from build123d import *

# Parameters (mm, degrees)
CROQUIS1_W              = 8.2
CROQUIS1_H              = 3
CROQUIS1_W_2            = 3
CROQUIS1_H_2            = 7.7
CROQUIS1_W_3            = 40
CROQUIS1_H_3            = 40
SALIENTE_EXTRUIR1_DEPTH = 3


with BuildPart() as part:
    # Croquis1 → Saliente-Extruir1 (new body)
    with BuildSketch(Plane.XY):
        Polygon((-20, 20), (-11.8, 20), (-11.8, 23), (-23, 23), (-23, 20), align=None)
        with Locations((0, 21.5)):
            Rectangle(CROQUIS1_W, CROQUIS1_H)
        Polygon((11.8, 20), (20, 20), (23, 20), (23, 23), (11.8, 23), align=None)
        with Locations((21.5, 7.95)):
            Rectangle(CROQUIS1_W_2, CROQUIS1_H_2)
        with Locations((21.5, -7.95)):
            Rectangle(CROQUIS1_W_2, CROQUIS1_H_2)
        Polygon((23, -20), (20, -20), (11.8, -20), (11.8, -23), (23, -23), align=None)
        with Locations((0, -21.5)):
            Rectangle(CROQUIS1_W, CROQUIS1_H)
        Polygon((-11.8, -23), (-11.8, -20), (-20, -20), (-23, -20), (-23, -23), align=None)
        with Locations((-21.5, 7.95)):
            Rectangle(CROQUIS1_W_2, CROQUIS1_H_2)
        Rectangle(CROQUIS1_W_3, CROQUIS1_H_3)
        with Locations((-21.5, -7.95)):
            Rectangle(CROQUIS1_W_2, CROQUIS1_H_2)
    extrude(amount=SALIENTE_EXTRUIR1_DEPTH)


solid = part.part
Can you work these out from the model? Positions are in its coordinate system, mm. A direction names the side the tool comes from. Coordinates: 2 decimals unless noted, no trailing zeros. Loops run counter-clockwise (first coordinate to the right, second up) from the corner with the lowest first, then second, coordinate; pieces in that order, holes last. Notation, with made-up numbers: (18.25, -9) - (24.25, -9) arc R13 ccw to (24.25, 12) - close; hole circle Ø6 at (44, -5). An arc over 180 degrees is marked (long way). Put each result on its own line as item: value. Start each with the question number.
Item 1: If we mould it in two halves opening along Y, with no side actions, what happens to faces 6 (the face through (0, 0, 3)), 7 (the face through (21, 20, 1)), 8 (the face through (-17, -23, 1))? For each: +Y half, -Y half, draft (parallel to the pull), parting line (faces both ways), or undercut.
Item 2: Suppose I cut it at A-A (y = 12.5). Please give me the cut outline in (x, z).
Item 3: For pin 1 (0.9 mm diameter, centred on y = -0.5, z = 2, fed in from +X); pin 2 (1.5 mm diameter, centred on y = 14, z = 1.5, fed in from -X), each with a flat end and sliding along its axis, tell me the tip position at first contact or that it passes through.
Item 4: If I drill on line 1 along X through (y, z) = (17, 2.15), over which ranges is the centre line in solid material (lowest first)?
Item 5: Which directions (+Z, -Z, +X, -X, +Y, -Y) give clear straight access to the entire face, cutting with the end or side of a thin tool? Please do faces 1 (the face through (4.1, -22, 1)), 2 (the face through (0, -23, 1)), 3 (the face through (-20, -16, 1)), 4 (the face through (21, -11.8, 1)), 5 (the face through (-11.8, 21, 1)).
Here are the results:
1. face 6: draft
1. face 7: undercut
1. face 8: -Y half
2. outline: (-20, 0) - (20, 0) - (20, 3) - (-20, 3) - close
3. pin 1: x = 20
3. pin 2: x = -20
4. line 1: -20 to 20
5. face 1: +Z, -Z, -Y
5. face 2: +Z, -Z, +X, -X, -Y
5. face 3: +Z, -Z, -X
5. face 4: +Z, -Z, +X
5. face 5: +Z, -Z, +Y
